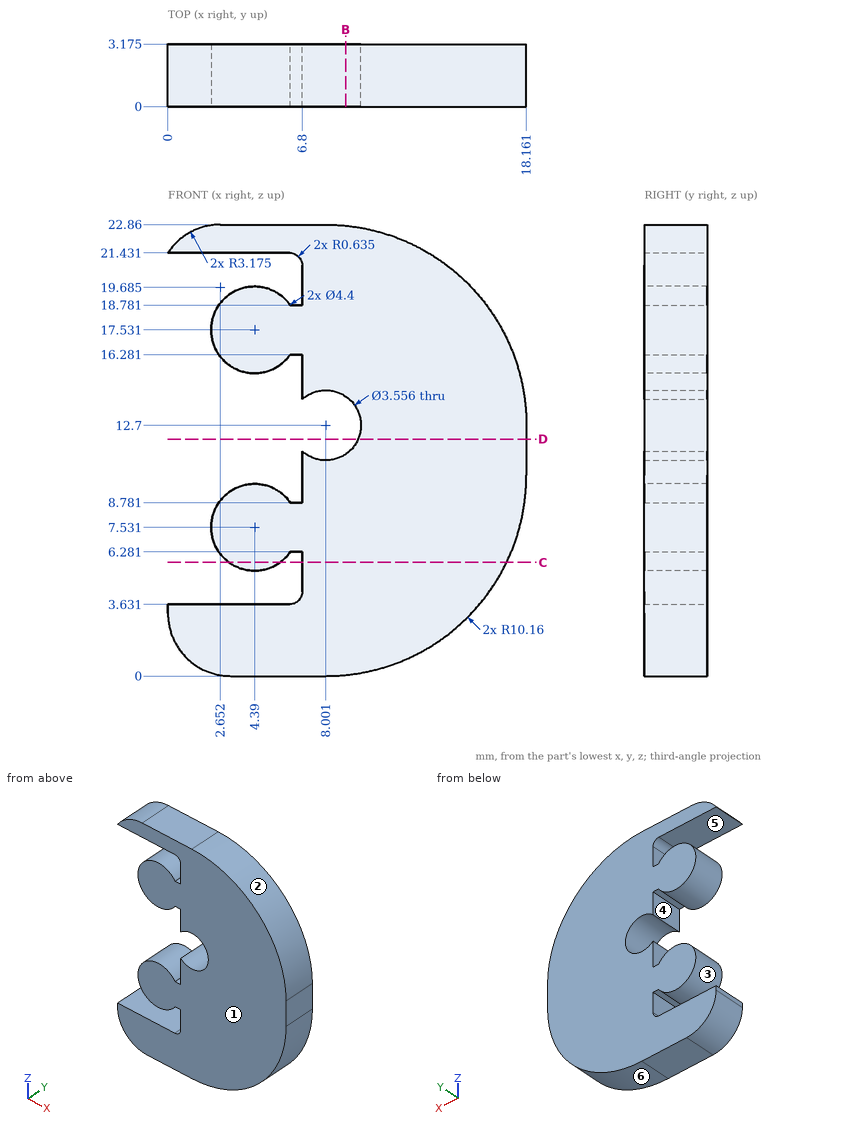
Here's the drawing with two shaded views (mm, measured from the low corner). I have some questions. A direction names the side the tool comes from. Round coordinates to 2 decimals unless told otherwise and drop trailing zeros. Loops run counter-clockwise (first coordinate to the right, second up) from the corner with the lowest first, then second, coordinate; pieces in that order, holes last.
Item 1: Suppose I cut it at C-C, the plane z = 5.75. Write out the boundary of the cut face in (x, y) (1 decimal).
Item 2: Which directions (+Z, -Z, +X, -X, +Y, -Y) give clear straight access to the entire face, cutting with the end or side of a thin tool? Please do the marked faces 4, 5 and 6.
Item 3: Please list where these lines run through material, in increasing order: L1, parallel to Z at x = 6.25, y = 3.05 (1 decimal); L2, parallel to Z at x = 4.5, y = 1; L3, parallel to Z at x = 8.5, y = 2.15.
Item 4: If we mould it in two halves opening along X, with no side actions, what happens to the marked faces 1, 2 and 3? For each: +X half, -X half, draft (parallel to the pull), parting line (faces both ways), or undercut.
Item 5: Suppose I cut it at B-B, the plane x = 9. Write out the boundary of the cut face in (y, z) (1 decimal).
Item 6: Will these pins go through, and if not, where does the flat tip stop? pin 1 Ø0.8 at (y, z) = (2.5, 10.5) entering from -X; pin 2 Ø1.8 at (y, z) = (1.5, 15.5) entering from -X; pin 3 Ø1 at (x, y) = (13, 2) entering from -Z; pin 4 Ø2 at (x, z) = (8.001, 12.7) entering from +Y.
Item 7: Suppose I cut it at D-D, the plane z = 12. Write out the boundary of the cut face in (x, y) (1 decimal), then the cut area to 3 significant figures.
Reported:
1. outline: (3.1, 0) - (5.7, 0) - (5.7, 3.2) - (3.1, 3.2) - close; (6.8, 0) - (17.2, 0) - (17.2, 3.2) - (6.8, 3.2) - close
2. face 4: +Y, -Y
2. face 5: -X, +Y, -Y
2. face 6: -Z, +X, +Y, -Y
3. L1: z = 0 to 3.6, 6.3 to 8.8, 16.3 to 18.8, 21.4 to 22.9
3. L2: z = 0 to 3.63, 5.33 to 9.73, 15.33 to 19.73, 21.43 to 22.86
3. L3: z = 0.01 to 10.99, 14.41 to 22.85
4. face 1: draft
4. face 2: +X half
4. face 3: undercut
5. outline: (0, 0) - (3.2, 0) - (3.2, 11.2) - (0, 11.2) - close; (0, 14.2) - (3.2, 14.2) - (3.2, 22.8) - (0, 22.8) - close
6. pin 1: stops at x = 6.8
6. pin 2: stops at x = 2.5
6. pin 3: stops at z = 1.05
6. pin 4: passes through
7. outline: (9.6, 0) - (18.2, 0) - (18.2, 3.2) - (9.6, 3.2) - close
7. area: 27.1 mm2
